Autodesk Fusion 360 part; units mm, degrees
sketch "Schizzo1" plane through (0, 0, 0) normal (0, 1, 0) x (1, 0, 0)
  line L0 (584, 0) -> (0, 0) construction
  line L1 (0, 0) -> (0, -20)
  line L2 (0, -20) -> (280, -300)
  line L3 (280, -300) -> (304, -300)
  line L4 (304, -300) -> (584, -20)
  line L5 (584, -20) -> (584, 0)
  line L6 (50.7107, 0) -> (270.7107, -220)
  line L7 (270.7107, -220) -> (313.2893, -220)
  line L8 (313.2893, -220) -> (533.2893, 0)
  line L9 (0, 0) -> (50.7107, 0)
  line L10 (533.2893, 0) -> (584, 0)
  line L11 (392.15, -211.85) -> (392.15, -200.15)
  line L12 (392.15, -200.15) -> (403.85, -200.15)
  line L13 (180.15, -200.15) -> (191.85, -200.15)
  line L14 (191.85, -200.15) -> (191.85, -211.85)
  line L15 (191.85, -200.15) -> (392.15, -200.15) construction
  dimension "d2" = 45
  dimension "d3" = 45
  dimension "d4" = 20
  dimension "d6" = 20
  dimension "d7" = 584
  dimension "d8" = 50
  dimension "d9" = 50
  dimension "d10" = 80
  dimension "d15" = 300
  dimension "d18" = 200.15
  dimension "d19" = 200.3
  dimension "d20" = 11.7
extrude "Estrusione1" add sketch "Schizzo1" along normal blind 4 contours L1 L2 L3 L4 L5 L6 L7 L8 L9 L10 L11 L12 L13 L14
component "Component" placed x (1, 0, 0) y (0, 1, 0) z (0, 0, 1) at (0, 0, 0)
equation "d18 = 200 mm + t"
equation "d19 = 200 mm + 2 * t"
The listing builds one solid part. Answer for the finished solid, in the listing's coordinates (mm). A direction names the side the tool comes from. Round coordinates to 2 decimals unless told otherwise and drop trailing zeros. Loops run counter-clockwise (first coordinate to the right, second up) from the corner with the lowest first, then second, coordinate; pieces in that order, holes last. Notation, with made-up numbers: M -33.75,10.5 L -19.75,10.5 A26 cw -19.75,48.5 Z; hole C 86.25,-16.75 d5. An arc over 180 degrees is marked long. Return JSON: item names as keys, results as strings.
Q1. Find section A-A, the plane y = 1.6. Determine the outline of the cut face in (x, z).
Results list:
{"outline": "M 0,0 L 50.71,0 L 270.71,220 L 313.29,220 L 533.29,0 L 584,0 L 584,20 L 403.85,200.15 L 392.15,200.15 L 392.15,211.85 L 304,300 L 280,300 L 191.85,211.85 L 191.85,200.15 L 180.15,200.15 L 0,20 Z"}
Q2. Which of the six approach directions +Z, -Z, +X, -X, +Y, -Y give full straight-line access (tool end or side, diameter ignored) to faces 1 (the face through (235, 2, 255)), 2 (the face through (159.17, 1.97, 108.46))?
Results list:
{"face 1": "+Z, -X, +Y, -Y", "face 2": "-Z, +Y, -Y"}
Q3. Find section D-D, the plane x = 67.5. Determine the outline of the cut face in (y, z), plus the area to 3 significant figures.
Results list:
{"outline": "M 0,16.79 L 4,16.79 L 4,87.5 L 0,87.5 Z", "area": "283 mm2"}
Q4. Each of these flat-tipped pins is pushed along its axis until it touches: pin 1 Ø1.2 at (y, z) = (2.5, 208.5) entering from -X; pin 2 Ø1.2 at (y, z) = (2, 206.5) entering from +X. Where does it stop, or does it pass through?
Results list:
{"pin 1": "stops at x = 191.85", "pin 2": "stops at x = 392.15"}
Q5. The mould has two halves that part along X. Classify faces 3 (the face through (89, 2, 109)), 4 (the face through (347, 2, 257)), 5 (the face through (421.75, 1.97, 111.54)): released by +X, released by -X, zero draft, split by the parting line, or undercut.
Results list:
{"face 3": "released by -X", "face 4": "released by +X", "face 5": "undercut"}
Q6. Find the intervals of material crossed by line 1 along X through (y, z) = (0.45, 174); line 2 along X through (y, z) = (1.5, 209); line 3 along Z through (x, y) = (289, 2.8), in increasing order. Write a range as from..to.
Results list:
{"line 1": "x = 154..224.71, 359.29..430", "line 2": "x = 191.85..259.71, 324.29..392.15", "line 3": "z = 220..300"}
Q7. Find section B-B, the plane z = 173. Determine the outline of the cut face in (x, y), plus the area to 3 significant figures.
Results list:
{"outline": "M 153,0 L 223.71,0 L 223.71,4 L 153,4 Z; M 360.29,0 L 431,0 L 431,4 L 360.29,4 Z", "area": "566 mm2"}
Q8. Find section C-C, the plane z = 271. Determine the outline of the cut face in (x, y).
Results list:
{"outline": "M 251,0 L 333,0 L 333,4 L 251,4 Z"}
